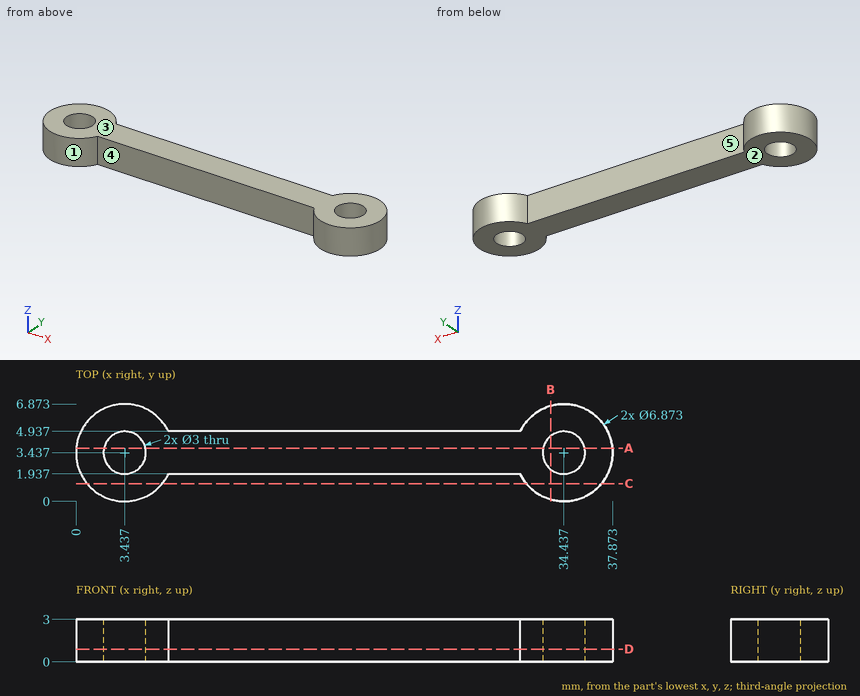
Job drawing, mm, ordinate dimensions from the low corner. One solid piece. A direction names the side the tool comes from. Round coordinates to 2 decimals unless told otherwise and drop trailing zeros. Write each loop counter-clockwise with the first axis right and the second up, starting at its lowest first coordinate (ties: lowest second). Pieces come first, ordered by that corner, then holes.
1) 3-axis set-ups, long thin cutter, end or side, ignore diameter. For the marked faces 3, 4 and 5: which of +Z, -Z, +X, -X, +Y, -Y reach the whole face in a straight line?
2) Pin check, flat tip, straight feed: pin 1 (1.5 mm diameter, centred on x = 22, z = 1, fed in from +Y). Stop position of the tip, or through.
3) Drill centre lines: probe 1 along X at (y, z) = (3.5, 2.45) (1 decimal); probe 2 along X at (y, z) = (4.75, 2.6) (1 decimal); probe 3 along Y at (x, z) = (18.5, 1). Where is each one in solid material? Low to high.
4) Band-saw the part on A-A, the plane y = 3.75. List the corners of the cut face in (x, z) (1 decimal).
5) Band-saw the part on D-D, the plane z = 0.9. List the corners of the cut face in (x, y) (1 decimal).
6) Band-saw the part on C-C, the plane y = 1.25. List the corners of the cut face in (x, z) (1 decimal), and give its area (3 significant figures).
7) Mould opens along X. For the marked faces 1 and 2 say: +X half, -X half, draft (parallel to the pull), parting line (faces both ways), or undercut.
8) Band-saw the part on B-B, the plane x = 33.5. List the corners of the cut face in (y, z) (1 decimal), and give its area (3 significant figures).
Ans:
1. face 3: +Z, +X, -X, +Y, -Y
1. face 4: +Z, -Z, -Y
1. face 5: +Z, -Z, +Y
2. pin 1: stops at y = 4.94
3. probe 1: x = 0 to 1.9, 4.9 to 32.9, 35.9 to 37.9
3. probe 2: x = 0.3 to 2.7, 4.2 to 33.7, 35.2 to 37.6
3. probe 3: y = 1.94 to 4.94
4. outline: (0, 0) - (2, 0) - (2, 3) - (0, 3) - close; (4.9, 0) - (33, 0) - (33, 3) - (4.9, 3) - close; (35.9, 0) - (37.9, 0) - (37.9, 3) - (35.9, 3) - close
5. outline: (6.5, 1.9) - (31.3, 1.9) arc R3.4 ccw (long way) to (31.3, 4.9) - (6.5, 4.9) arc R3.4 ccw (long way) to start; hole circle Ø3 at (3.4, 3.4); hole circle Ø3 at (34.4, 3.4)
6. outline: (0.8, 0) - (6.1, 0) - (6.1, 3) - (0.8, 3) - close; (31.8, 0) - (37.1, 0) - (37.1, 3) - (31.8, 3) - close
6. area: 31.8 mm2
7. face 1: undercut
7. face 2: draft
8. outline: (0.1, 0) - (2.3, 0) - (2.3, 3) - (0.1, 3) - close; (4.6, 0) - (6.7, 0) - (6.7, 3) - (4.6, 3) - close
8. area: 12.8 mm2
